```python
from build123d import *

# Parameters (mm, degrees)
F0_W     = 152.4
F0_H     = 19.05
F1_DEPTH = 25.4
F2_W     = 66.552096
F2_H     = 7.88629
F3_DEPTH = 6.35


with BuildPart() as f1:
    # F0 (on Front) → F1 (new body)
    with BuildSketch(Plane.XZ):
        Rectangle(F0_W, F0_H)
    extrude(amount=F1_DEPTH)

    # F2 (on face) → F3 (join)
    with BuildSketch(Plane.XY.offset(9.525)):
        with Locations((0, -12.7)):
            Rectangle(F2_W, F2_H)
    extrude(amount=F3_DEPTH)


solid = f1.part
```
Geometry check sheet. Reference: the model listing, model coordinates, mm. A direction names the side the tool comes from. Coordinates: 2 decimals unless noted, no trailing zeros. Order: outer loops, then holes, each group sorted by start corner. A loop starts at its lowest first (then second) coordinate and runs counter-clockwise, first axis right, second up. Notation, with made-up numbers: (30.5, 16.25) - (86.5, 16.25) arc R20 cw to (86.5, 35.25) - close; hole circle Ø7 at (-10, -15). An arc over 180 degrees is marked (long way). Answer as a JSON object with one key per item and string values. Group by question number.
Item 1: Sectioned sample at D-D, the plane y = -22. Record the cut outline in (x, z) (3 decimals), and give its area (3 significant figures).
Item 2: Sectioned sample at A-A, the plane y = -12.5. Record the cut outline in (x, z) (3 decimals), and give its area (3 significant figures).
Item 3: Scan lines: probe 1 along X at (y, z) = (-9, 12.25); probe 2 along Z at (x, y) = (23, -1.75) (3 decimals); probe 3 along Y at (x, z) = (-6, 14). Record each from-to range of solid material in increasing order.
Item 4: Depth check by flat-ended pin: pin 1 Ø2 at (x, y) = (48.5, -2.5) entering from +Z (3 decimals); pin 2 Ø3 at (x, z) = (11.5, 13) entering from +Y; pin 3 Ø1.9 at (x, z) = (16.5, 13) entering from -Y. Enter the tip coordinate at first touch or a pass-through.
Item 5: Sectioned sample at C-C, the plane z = 12. Record the cut outline in (x, y), and give its area (3 significant figures).
Item 6: Sectioned sample at B-B, the plane x = -18. Record the cut outline in (y, z) (3 decimals), and give its area (3 significant figures).
Item 7: Tool access check on faces 1 (the face through (-33.276, -13, 13)), 2 (the face through (33.276, -13, 13)), 3 (the face through (0, -8.757, 13)). Record the directions out of +Z, -Z, +X, -X, +Y, -Y that give a thin tool (end or side, any length) a straight path to the whole face; none if there is none.
Resolved:
{
 "1": {"outline": "(-76.2, -9.525) - (76.2, -9.525) - (76.2, 9.525) - (-76.2, 9.525) - close", "area": "2,900 mm^2"},
 "2": {"outline": "(-76.2, -9.525) - (76.2, -9.525) - (76.2, 9.525) - (33.276, 9.525) - (33.276, 15.875) - (-33.276, 15.875) - (-33.276, 9.525) - (-76.2, 9.525) - close", "area": "3,330 mm^2"},
 "3": {"probe 1": "-33.28 to 33.28", "probe 2": "-9.525 to 9.525", "probe 3": "-16.64 to -8.76"},
 "4": {"pin 1": "z = 9.525", "pin 2": "y = -8.76", "pin 3": "y = -16.64"},
 "5": {"outline": "(-33.28, -16.64) - (33.28, -16.64) - (33.28, -8.76) - (-33.28, -8.76) - close", "area": "525 mm^2"},
 "6": {"outline": "(-25.4, -9.525) - (0, -9.525) - (0, 9.525) - (-8.757, 9.525) - (-8.757, 15.875) - (-16.643, 15.875) - (-16.643, 9.525) - (-25.4, 9.525) - close", "area": "534 mm^2"},
 "7": {"face 1": "+Z, -X, +Y, -Y", "face 2": "+Z, +X, +Y, -Y", "face 3": "+Z, +X, -X, +Y"}
}
